Part model, mm, in its own coordinate system. A direction names the side the tool comes from. Give positions to 0.01 mm unless a question says otherwise; leave off trailing zeros. Loops run counter-clockwise (first coordinate to the right, second up) from the corner with the lowest first, then second, coordinate; pieces in that order, holes last. Notation, with made-up numbers: M 87.5,68 L 98.5,68 A20 cw 98.5,85 Z; hole C 7,41.25 d2. An arc over 180 degrees is marked long. Answer in a Markdown table with one row per item.
from build123d import *

# Parameters (mm, degrees)
CUT_EXTRUDE1_REACH      = 142.114
CUT_EXTRUDE1_END_RADIUS = 19.05
SKETCH3_R               = 6.35


with BuildPart() as part:
    # Sketch1 → Revolve1 (revolve)
    with BuildSketch(Plane.XY, mode=Mode.PRIVATE) as revolve1_sk:
        with BuildLine():
            Line((-137.5, 0), (137.5, 0))
            Line((137.5, 0), (137.5, 7.747))
            add(Edge.make_bspline(
                [(119.602, 16.764), (126.446685513, 16.474787936), (132.251729161, 15.730759902), (137.5, 12.322795174), (137.5, 7.747)],
                knots=[0, 0, 0, 0, 0.656247862, 1, 1, 1, 1], degree=3))
            Line((119.602, 16.764), (65.5, 19.05))
            Line((65.5, 19.05), (-14.564, 19.05))
            add(Edge.make_bspline(
                [(-91.78, 17.399), (-84.901336541, 18.220618135), (-60.549292723, 10.012805319), (-35.82944709, 19.05), (-14.564, 19.05)],
                knots=[0, 0, 0, 0, 0.244238151, 1, 1, 1, 1], degree=3))
            Line((-91.78, 17.399), (-137.5, 11.938))
            Line((-137.5, 11.938), (-137.5, 0))
        make_face()
    revolve(revolve1_sk.sketch.rotate(Axis((-137.5, 0, 0), (1, 0, 0)), 180), axis=Axis((-137.5, 0, 0), (1, 0, 0)))

    # Cut-Extrude1: up to this cylinder (the profile starts inside it)
    cut_extrude1_end = Plane(origin=(12.36, 0, 0), z_dir=(-1, 0, 0)) * Cylinder(CUT_EXTRUDE1_END_RADIUS, 323.328, mode=Mode.PRIVATE)
    # Sketch3 → Cut-Extrude1 (cut, up to the surface)
    with BuildSketch(Plane(origin=(0, 0, 0), x_dir=(1, 0, 0), z_dir=(0, 1, 0)), mode=Mode.PRIVATE) as cut_extrude1_sk1:
        with Locations(Location((12.36, 0, 0), (0, 0, 90))):
            Circle(SKETCH3_R)
    cut_extrude1_tool1 = extrude(cut_extrude1_sk1.sketch, amount=CUT_EXTRUDE1_REACH, mode=Mode.PRIVATE) & cut_extrude1_end
    add(cut_extrude1_tool1.solids().sort_by_distance((12.36, 0, 0))[0], mode=Mode.SUBTRACT)


solid = part.part
(1) Which spindle directions (+Z, -Z, +X, -X, +Y, -Y) get a long thin tool onto all of the face, cutting with end or side? Do faces 1 (the face through (92.172, 17.906, -0.788)), 2 (the face through (17.994, 9.399, -2.93)). Say none if no direction does.
Recorded:
| item | result |
|---|---|
| face 1 | +X |
| face 2 | +Y |
(2) Saw through at B-B (x = 108.5). Write the cut outline in (y, z), plus the area to 3 significant figures.
Recorded:
| item | result |
|---|---|
| outline | C 0,0 d34.47 |
| area | 933 mm^2 |
(3) Saw through at A-A (x = 26). Write the cut outline in (y, z), plus the area to 3 significant figures.
Recorded:
| item | result |
|---|---|
| outline | C 0,0 d38.1 |
| area | 1,140 mm^2 |
(4) Drill centre lines: line 1 along X through (y, z) = (3.5, -1.5); line 2 along X through (y, z) = (11.5, 0); line 3 along X through (y, z) = (6, -6.5). Where is each one in solid material? Low to high.
Recorded:
| item | result |
|---|---|
| line 1 | x = -137.5 to 6.19, 18.53 to 137.5 |
| line 2 | x = -137.5 to 6.01, 18.71 to 136.88 |
| line 3 | x = -137.5 to 137.46 |
(5) Pin check, flat tips, straight feed: pin 1 Ø1 at (x, y) = (-19.5, 12.5) entering from -Z; pin 2 Ø8 at (x, z) = (-106, 1.5) entering from -Y; pin 3 Ø4 at (x, y) = (72.5, 12) entering from +Z. Stop position of each tip, or through.
Recorded:
| item | result |
|---|---|
| pin 1 | stops at z = -14.65 |
| pin 2 | stops at y = -16.16 |
| pin 3 | stops at z = 15.87 |
(6) Pull direction X, two halves, no side cores. Call faces 3 (the face through (12, 0, 0)), 4 (the face through (-114.96, -6.75, 12.98)), 5 (the face through (137.5, 0, 0)): +X half, -X half, draft (parallel to the pull), parting line (faces both ways), or undercut.
Recorded:
| item | result |
|---|---|
| face 3 | undercut |
| face 4 | -X half |
| face 5 | +X half |
